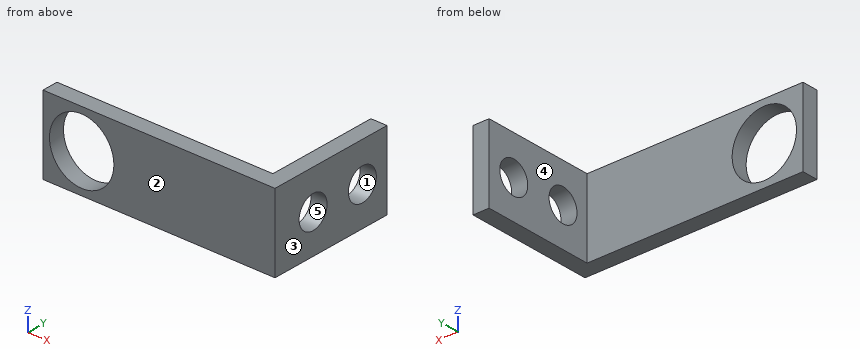
from build123d import *

# Parameters (mm, degrees)
SKETCH1_W                    = 23.8125
SKETCH1_H                    = 7.62
BOSS_EXTRUDE1_DEPTH          = 1.5875
SKETCH1_4_W                  = 1.5875
SKETCH1_4_H                  = 7.62
BOSS_EXTRUDE2_DEPTH          = 12.7
F_1_4_0_25_DIAMETER_HOLE1_D  = 6.35
CUT_EXTRUDE2_DEPTH           = 29.752600861
CUT_EXTRUDE2_DEPTH_BACK      = 1.5875
F_1_8_0_125_DIAMETER_HOLE1_D = 3.175


with BuildPart() as part:
    # Sketch1 → Boss-Extrude1 (new body)
    with BuildSketch(Plane(origin=(0, 0, 0), x_dir=(1, 0, 0), z_dir=(0, 1, 0))):
        with Locations((-13.49375, 3.81)):
            Rectangle(SKETCH1_W, SKETCH1_H)
    extrude(amount=BOSS_EXTRUDE1_DEPTH)

    # Sketch1<4> → Boss-Extrude2 (add)
    with BuildSketch(Plane(origin=(0, 0, 0), x_dir=(1, 0, 0), z_dir=(0, 1, 0))):
        with Locations((-0.79375, 3.81)):
            Rectangle(SKETCH1_4_W, SKETCH1_4_H)
    extrude(amount=BOSS_EXTRUDE2_DEPTH)

    # 1/4 (0.25) Diameter Hole1 (through all)
    with Locations(Plane(origin=(0, 0, 0), x_dir=(-1, 0, 0), z_dir=(0, -1, 0))):
        with Locations((19.05, 3.81)):
            Hole(F_1_4_0_25_DIAMETER_HOLE1_D / 2)

    # Sketch7 → Cut-Extrude2 (cut, two sides: drawn at the far end of the back side and taken through both)
    with BuildSketch(Plane(origin=(0, 1.5875, 0), x_dir=(1, 0, 0), z_dir=(0, 1, 0)).offset(-CUT_EXTRUDE2_DEPTH_BACK)):
        Polygon((-22.86, 65.813111541), (-22.86, 7.62), (-22.86, 0), (-22.86, -58.193111541), (-139.246223082, -58.193111541), (-139.246223082, 65.813111541), align=None)
    extrude(amount=CUT_EXTRUDE2_DEPTH + CUT_EXTRUDE2_DEPTH_BACK, mode=Mode.SUBTRACT)

    # 1/8 (0.125) Diameter Hole1 (through all)
    with Locations(Plane.ZY.offset(1.5875)):
        with Locations((-3.834673101, 9.906), (-3.834673101, 4.318)):
            Hole(F_1_8_0_125_DIAMETER_HOLE1_D / 2)


solid = part.part
Could you check a few things on this model? Use its own coordinates, in mm. Face numbers are marked on the shaded views. A direction names the side the tool comes from. Give positions to 0.01 mm unless a question says otherwise; leave off trailing zeros. Order: outer loops, then holes, each group sorted by start corner. A loop starts at its lowest first (then second) coordinate and runs counter-clockwise, first axis right, second up. Notation, with made-up numbers: (44.5, -6.5) - (100.5, -6.5) arc R26 cw to (100.5, 25.5) - close; hole circle Ø2 at (-31, 59.25). An arc over 180 degrees is marked (long way). One line per item, written item: value. Start each with the question number.
1. Thinking about a two-plate mould opening in Y: for the marked faces 1, 2 and 3, which applies, +Y half, -Y half, draft (parallel to the pull), parting line (faces both ways), or undercut?
2. Imagine slicing it at D-D on z = -3.81. List the corners of the cut face in (x, y) for me (1 decimal).
3. Imagine slicing it at C-C on y = 11. List the corners of the cut face in (x, z) for me.
4. Imagine slicing it at B-B on z = -1.5. List the corners of the cut face in (x, y) for me, plus the area to 3 significant figures.
5. For the marked faces 4 and 5, which set-ups out of +Z, -Z, +X, -X, +Y, -Y let a thin tool reach every point of the face, with its end or its side?
6. For P1, Ø3, axis at y = 4.32, z = -3.83, coming from the -X side; P2, Ø2, axis at y = 8, z = -6.5, coming from the -X side, each with a flat end and sliding along its axis, tell me the tip position at first contact or that it passes through.
7. If I drill on probe 1 along Y at (x, z) = (-1.5, -3.75); probe 2 along Z at (x, y) = (-19.05, 1.05) (3 decimals); probe 3 along Y at (x, z) = (-15.25, -5.25), over which ranges is the centre line in solid material (lowest first)?
8. Imagine slicing it at A-A on x = -19.05. List the corners of the cut face in (y, z) for me (1 decimal).
Values:
1. face 1: undercut
1. face 2: -Y half
1. face 3: draft
2. outline: (-22.9, 0) - (-22.2, 0) - (-22.2, 1.6) - (-22.9, 1.6) - close; (-15.9, 0) - (0, 0) - (0, 2.7) - (-1.6, 2.7) - (-1.6, 1.6) - (-15.9, 1.6) - close; (-1.6, 5.9) - (0, 5.9) - (0, 8.3) - (-1.6, 8.3) - close; (-1.6, 11.5) - (0, 11.5) - (0, 12.7) - (-1.6, 12.7) - close
3. outline: (-1.59, -7.62) - (0, -7.62) - (0, -4.99) - (-1.59, -4.99) - close; (-1.59, -2.68) - (0, -2.68) - (0, 0) - (-1.59, 0) - close
4. outline: (-22.86, 0) - (-21.23, 0) - (-21.23, 1.59) - (-22.86, 1.59) - close; (-16.87, 0) - (0, 0) - (0, 12.7) - (-1.59, 12.7) - (-1.59, 1.59) - (-16.87, 1.59) - close
4. area: 47.0 mm²
5. face 4: +Z, -Z, -X, +Y
5. face 5: +X, -X
6. P1: through
6. P2: x = -1.59
7. probe 1: 0 to 2.73, 5.9 to 8.32, 11.49 to 12.7
7. probe 2: -7.62 to -6.985, -0.635 to 0
7. probe 3: 0 to 1.59
8. outline: (0, -7.6) - (1.6, -7.6) - (1.6, -7) - (0, -7) - close; (0, -0.6) - (1.6, -0.6) - (1.6, 0) - (0, 0) - close
